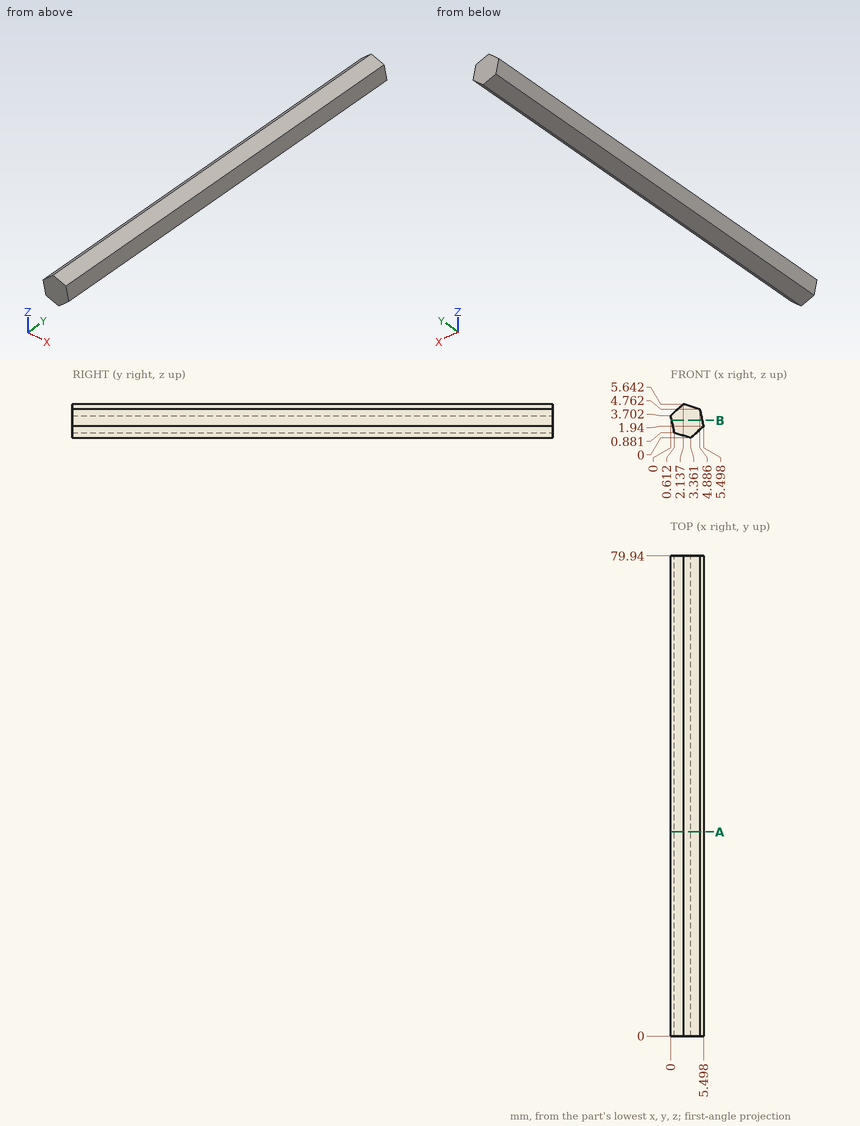
Drawing for the job (mm, zero at the part's lowest x, y, z). Coordinates: 2 decimals unless noted, no trailing zeros. Write each loop counter-clockwise with the first axis right and the second up, starting at its lowest first coordinate (ties: lowest second). Pieces come first, ordered by that corner, then holes. Notation, with made-up numbers: (-0.75, 32.5) -> (39.25, 32.5) arc R21 cw to (39.25, 36.5) -> close; hole circle Ø9 at (73.25, 4.5). An arc over 180 degrees is marked (long way). One line per item, written item: value. Start each with the question number.
1) Slice it at B-B on z = 2.9. Write the cut outline in (x, y).
2) Slice it at A-A on y = 34. Write the cut outline in (x, z).
3) Probe probe 1 along Z at (x, y) = (4.8, 46) (1 decimal); probe 2 along Z at (x, y) = (2.2, 27); probe 3 along X at (y, z) = (74.5, 2.7). List the from-to ranges inside material, lowest first.
4) Flat gauge pins, fed straight in: pin 1 Ø1 at (x, y) = (4.5, 59) entering from +Z (1 decimal); pin 2 Ø1.5 at (y, z) = (47, 3.5) entering from +X; pin 3 Ø3 at (x, y) = (1.5, 17.5) entering from -Z (1 decimal). Where does each tip first touch, or does it go through?
Answers follow:
1. outline: (0.17, 0) -> (5.29, 0) -> (5.29, 79.94) -> (0.17, 79.94) -> close
2. outline: (0, 3.7) -> (0.61, 0.88) -> (3.36, 0) -> (5.5, 1.94) -> (4.89, 4.76) -> (2.14, 5.64) -> close
3. probe 1: 1.3 to 4.8
3. probe 2: 0.37 to 5.62
3. probe 3: 0.22 to 5.33
4. pin 1: z = 5
4. pin 2: x = 5.32
4. pin 3: z = 0.1
